Input: part model. Units: mm. Frame: model coordinates. Round coordinates to 2 decimals unless told otherwise and drop trailing zeros. Order: outer loops, then holes, each group sorted by start corner. A loop starts at its lowest first (then second) coordinate and runs counter-clockwise, first axis right, second up. Notation, with made-up numbers: (-39, 72.25) -> (-4, 72.25) arc R21 ccw to (-4, 88.25) -> close; hole circle Ø9 at (-40, 60). An arc over 180 degrees is marked (long way). Use a Markdown table: item, result.
from build123d import *

# Parameters (mm, degrees)
PRESS_SOVE_SAG_1_START = 120
PRESS_SOVE_SAG_1_DEPTH = 1850


with BuildPart() as part:
    # Sketch1 → PRESS_sove_sag_1 (new body)
    with BuildSketch(Plane(origin=(0, 0, 0), x_dir=(1, 0, 0), z_dir=(0, 1, 0)).offset(PRESS_SOVE_SAG_1_START)):
        Polygon((700, -40), (700, -38.5), (671.5, -38.5), (671.5, 0), (670, 0), (670, -40), align=None)
    extrude(amount=PRESS_SOVE_SAG_1_DEPTH)


solid = part.part
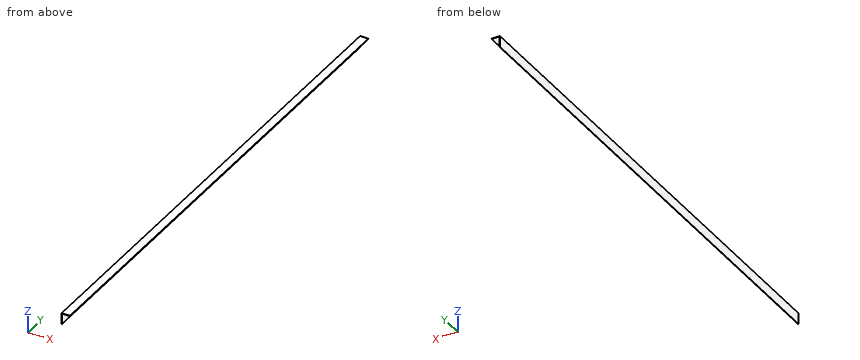
1) Pin query (flat end, axial travel): pin 1 Ø4 at (y, z) = (955, 19) entering from +X; pin 2 Ø12 at (x, y) = (684, 463.5) entering from -Z; pin 3 Ø10 at (x, z) = (678, 28.5) entering from +Y. Return the tip coordinate at first contact, or that it passes through.
Results found:
| item | result |
|---|---|
| pin 1 | stops at x = 671.5 |
| pin 2 | stops at z = 38.5 |
| pin 3 | passes through |
2) Cut plane A-A on y = 1564.5. Return loops of the section in (x, z).
Results found:
| item | result |
|---|---|
| outline | (670, 0) -> (671.5, 0) -> (671.5, 38.5) -> (700, 38.5) -> (700, 40) -> (670, 40) -> close |
3) Cut plane C-C on z = 15. Return loops of the section in (x, y), and give its area (4 significant figures).
Results found:
| item | result |
|---|---|
| outline | (670, 120) -> (671.5, 120) -> (671.5, 1970) -> (670, 1970) -> close |
| area | 2,775 mm² |
4) Cut plane B-B on x = 694.5. Return loops of the section in (y, z).
Results found:
| item | result |
|---|---|
| outline | (120, 38.5) -> (1970, 38.5) -> (1970, 40) -> (120, 40) -> close |
5) Line query: L1, parallel to X at y = 700.5, z = 13.5; L2, parallel to Z at x = 697, y = 1458. Output: solid intervals per line, ascending. Write a range as [from, to].
Results found:
| item | result |
|---|---|
| L1 | x = [670, 671.5] |
| L2 | z = [38.5, 40] |
